The drawing under review shows one solid part. Ordinate dimensions are in mm from its lowest x, y, z. A direction names the side the tool comes from. Round coordinates to 2 decimals unless told otherwise and drop trailing zeros. Order: outer loops, then holes, each group sorted by start corner. A loop starts at its lowest first (then second) coordinate and runs counter-clockwise, first axis right, second up. Notation, with made-up numbers: (-16, 11) -> (15, 11) arc R25 ccw to (15, 31) -> close; hole circle Ø10 at (-36, 83). An arc over 180 degrees is marked (long way). Use a Markdown table: item, result. Add a question column.
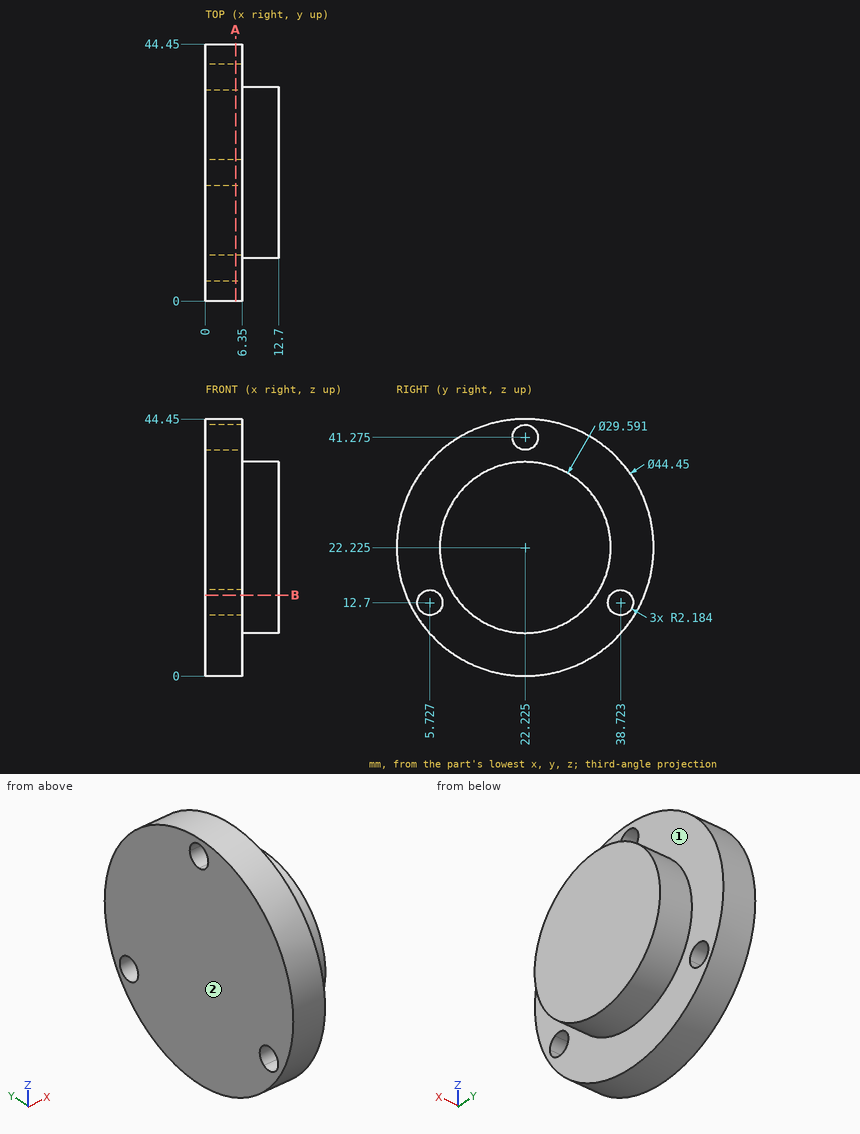
Q1. Add section B-B, the plane z = 14. Give the boundary of the cut face in (x, y), then the cut area to 3 significant figures.
Q2. Add section A-A, the plane x = 5.25. Give the number of separate pieces and of enclosed holes in the cut face, then the cut area to 3 significant figures.
Q3. For pin 1 (2 mm diameter, centred on x = 6.5, y = 10.5, fed in from +Z) (1 decimal); pin 2 (2 mm diameter, centred on x = 6.5, y = 15.5, fed in from -Z); pin 3 (1 mm diameter, centred on x = 2.5, y = 14.5, fed in from +Z), all flat-tipped, find the tip position at first contact; note any pin that passes through.
Q4. To check wall thickness, follow line 1 along X through (y, z) = (23.5, 38.5); line 2 along Y through (x, z) = (1.75, 8.5) (1 decimal); line 3 along Y through (x, z) = (11.75, 22). State the ranges of each line that lie inside material, in increasing order.
Q5. For the marked faces 1 and 2, list the 3-axis set-ups (+Z, -Z, +X, -X, +Y, -Y) from which the entire face can be reached by the end or side of a thin tool; tool diameter is ignored.
Return value:
| question | item | result |
|---|---|---|
| 1 | outline | (0, 1.58) -> (6.35, 1.58) -> (6.35, 3.97) -> (0, 3.97) -> close; (0, 7.48) -> (6.35, 7.48) -> (6.35, 9.93) -> (12.7, 9.93) -> (12.7, 34.52) -> (6.35, 34.52) -> (6.35, 36.97) -> (0, 36.97) -> close; (0, 40.48) -> (6.35, 40.48) -> (6.35, 42.87) -> (0, 42.87) -> close |
| 1 | area | 374 mm² |
| 2 | separate pieces | 1 |
| 2 | enclosed holes | 3 |
| 2 | area | 1,510 mm² |
| 3 | pin 1 | z = 41.7 |
| 3 | pin 2 | z = 0.75 |
| 3 | pin 3 | z = 43.24 |
| 4 | line 1 | 0 to 6.35 |
| 4 | line 2 | 4.7 to 39.7 |
| 4 | line 3 | 7.43 to 37.02 |
| 5 | face 1 | +X |
| 5 | face 2 | +Z, -Z, -X, +Y, -Y |
